```python
from build123d import *

# Parameters (mm, degrees)
F0_W     = 50
F0_H     = 50
F1_DEPTH = 125
F2_W     = 90
F2_H     = 30
F3_DEPTH = 50
F5_DEPTH = 125
F6_D     = 10.8
F6_DEPTH = 15
F6_TIP   = 3.2446473427
F7_SIZE  = 5


with BuildPart() as f1:
    # F0 (on Front) → F1 (new body)
    with BuildSketch(Plane.XZ):
        Rectangle(F0_W, F0_H)
    extrude(amount=F1_DEPTH)

    # F2 (on face) → F3 (cut)
    with BuildSketch(Plane.YZ.offset(25)):
        with Locations((-60, 10)):
            Rectangle(F2_W, F2_H)
    extrude(amount=-F3_DEPTH, mode=Mode.SUBTRACT)

    # F4 (on face) → F5 (cut)
    with BuildSketch(Plane(origin=(0, 0, 0), x_dir=(-1, 0, 0), z_dir=(0, 1, 0))):
        Polygon((-12.5, -15), (-12.5, -25), (12.5, -25), (12.5, -15), (7.5, -15), (7.5, -5), (-7.5, -5), (-7.5, -15), align=None)
    extrude(amount=-F5_DEPTH, mode=Mode.SUBTRACT)

    # F6
    with Locations(Plane(origin=(0, 0, 0), x_dir=(-1, 0, 0), z_dir=(0, 1, 0))):
        with Locations((0, 10)):
            Hole(F6_D / 2, depth=F6_DEPTH)
            with Locations((0, 0, -(F6_DEPTH + F6_TIP / 2))):  # 118° drill point
                Cone(0, F6_D / 2, F6_TIP, mode=Mode.SUBTRACT)

    # F7
    f7_edges = [f1.edges().sort_by_distance(p)[0] for p in [
        (0, -125, 25),
    ]]
    chamfer(f7_edges, length=F7_SIZE)


solid = f1.part
```
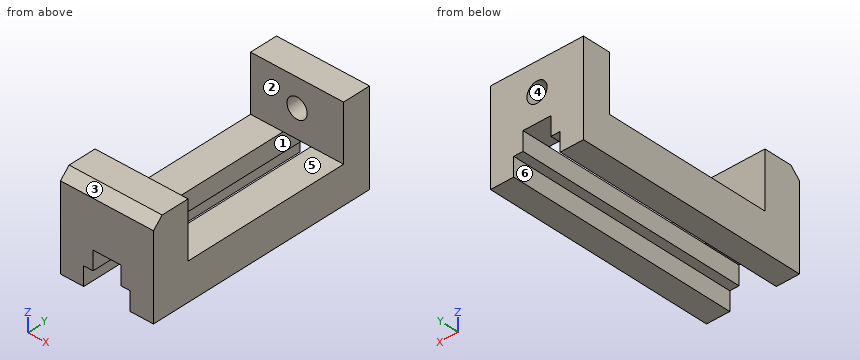
Part model, mm, in its own coordinate system. Face numbers are marked on the shaded views. A direction names the side the tool comes from. Coordinates: 2 decimals unless noted, no trailing zeros. Order: outer loops, then holes, each group sorted by start corner. A loop starts at its lowest first (then second) coordinate and runs counter-clockwise, first axis right, second up. Notation, with made-up numbers: (28.5, -6.5) - (77.5, -6.5) arc R7 cw to (77.5, 1.5) - close; hole circle Ø1 at (62, 37). An arc over 180 degrees is marked (long way). Return JSON: item names as keys, results as strings. Group by question number.
Item 1: Pull direction Y, two halves, no side cores. Call the marked faces 1, 2 and 3: pulls with the +Y half, pulls with the -Y half, needs draft (parallel to the pull), parting line crosses it, or undercut.
Item 2: Cut at A-A (x = 0). List the corners of the cut face in (y, z), plus the area to 4 significant figures.
Item 3: Drill centre lines: probe 1 along Z at (x, y) = (0, -7); probe 2 along Y at (x, z) = (-16.5, 15); probe 3 along X at (y, z) = (-61.5, -11.5). Where is each one in solid material? Low to high. Write a range as from..to.
Item 4: Which spindle directions (+Z, -Z, +X, -X, +Y, -Y) get a long thin tool onto all of the face, cutting with end or side? Do the marked faces 4, 5 and 6. Say none if no direction does.
Item 5: Pin check, flat tips, straight feed: pin 1 (10 mm diameter, centred on x = -1.5, y = -50, fed in from +Z); pin 2 (1.5 mm diameter, centred on x = -11, y = -70, fed in from -Z); pin 3 (14 mm diameter, centred on x = -13, y = -45, fed in from +Z); pin 4 (7.5 mm diameter, centred on x = -1.5, y = -8.5, fed in from -Z). Stop position of each tip, or through.
Item 6: Cut at D-D (x = -20). List the corners of the cut face in (y, z).
Item 7: Cut at C-C (z = 10). List the corners of the cut face in (x, y), plus the area to 3 significant figures.
Item 8: Cut at B-B (y = -24). List the corners of the cut face in (x, z).
Check values:
{
 "1": {"face 1": "needs draft", "face 2": "undercut", "face 3": "pulls with the -Y half"},
 "2": {"outline": "(-125, -5) - (-105, -5) - (-105, 25) - (-120, 25) - (-125, 20) - close; (-15, -5) - (0, -5) - (0, 4.6) - (-15, 4.6) - close; (-15, 15.4) - (0, 15.4) - (0, 25) - (-15, 25) - close", "area": "875.5 mm2"},
 "3": {"probe 1": "z = -5..4.6, 15.4..25", "probe 2": "y = -125..-105, -15..0", "probe 3": "x = -25..-7.5, 7.5..25"},
 "4": {"face 4": "+Y", "face 5": "+Z, +X, -X", "face 6": "-Z, +Y, -Y"},
 "5": {"pin 1": "passes through", "pin 2": "stops at z = -15", "pin 3": "stops at z = -5", "pin 4": "stops at z = -5"},
 "6": {"outline": "(-125, -25) - (0, -25) - (0, 25) - (-15, 25) - (-15, -5) - (-105, -5) - (-105, 25) - (-120, 25) - (-125, 20) - close"},
 "7": {"outline": "(-25, -125) - (25, -125) - (25, -105) - (-25, -105) - close; (-25, -15) - (-5.4, -15) - (-5.4, 0) - (-25, 0) - close; (5.4, -15) - (25, -15) - (25, 0) - (5.4, 0) - close", "area": "1,590 mm2"},
 "8": {"outline": "(-25, -25) - (-12.5, -25) - (-12.5, -15) - (-7.5, -15) - (-7.5, -5) - (-25, -5) - close; (7.5, -15) - (12.5, -15) - (12.5, -25) - (25, -25) - (25, -5) - (7.5, -5) - close"}
}
